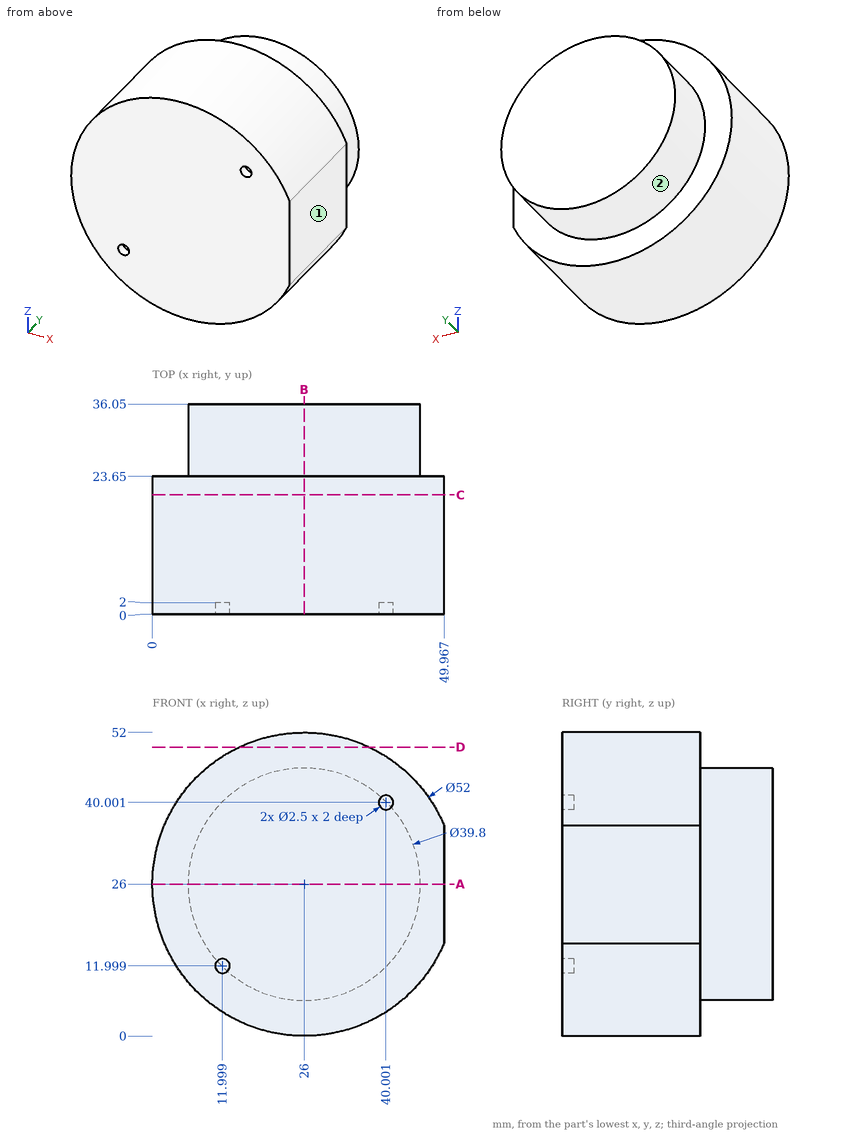
The drawing under review shows one solid part. Ordinate dimensions are in mm from its lowest x, y, z. A direction names the side the tool comes from. Coordinates: 2 decimals unless noted, no trailing zeros. Order: outer loops, then holes, each group sorted by start corner. A loop starts at its lowest first (then second) coordinate and runs counter-clockwise, first axis right, second up. Notation, with made-up numbers: (-34, -22.5) -> (-19, -22.5) arc R32 ccw to (-19, 16.5) -> close; hole circle Ø6 at (-3, 18.5). An arc over 180 degrees is marked (long way). Use CSV: the item, a comma, the result in double quotes. Start each with the question number.
Item 1: Insertion check: pin 1 (5 mm diameter, centred on x = 9.5, y = 19, fed in from +Z); pin 2 (10 mm diameter, centred on x = 40, y = 32.5, fed in from +Z); pin 3 (12 mm diameter, centred on y = 29, z = 45, fed in from -X). Each pin has a flat end and moves straight along its axis. Give the tip position at first contact, or say it passes through.
Item 2: We need section A-A, the plane z = 26. Give the boundary of the cut face in (x, y), then the cut area to 3 significant figures.
Item 3: Wall thickness on probe 1 along X at (y, z) = (17.5, 36); probe 2 along Y at (x, z) = (34, 6); probe 3 along X at (y, z) = (6, 26): over which ranges is each line inside the solid? List them lowest first.
Item 4: For the marked faces 1 and 2, list the 3-axis set-ups (+Z, -Z, +X, -X, +Y, -Y) from which the entire face can be reached by the end or side of a thin tool; tool diameter is ignored.
Item 5: We need section B-B, the plane x = 26. Give the boundary of the cut face in (y, z), then the cut area to 3 significant figures.
Item 6: We need section D-D, the plane z = 49.5. Give the boundary of the cut face in (x, y).
Item 7: We need section C-C, the plane y = 20.5. Give the boundary of the cut face in (x, z), then the cut area to 3 significant figures.
Derived:
1,pin 1,"stops at z = 47.91"
1,pin 2,"stops at z = 43.75"
1,pin 3,"stops at x = 5.73"
2,outline,"(0, 0) -> (49.97, 0) -> (49.97, 23.65) -> (45.9, 23.65) -> (45.9, 36.05) -> (6.1, 36.05) -> (6.1, 23.65) -> (0, 23.65) -> close"
2,area,"1,680 mm^2"
3,probe 1,"x = 2 to 49.97"
3,probe 2,"y = 0 to 23.65"
3,probe 3,"x = 0 to 49.97"
4,face 1,"+Z, -Z, +X, +Y, -Y"
4,face 2,"+Y"
5,outline,"(0, 0) -> (23.65, 0) -> (23.65, 6.1) -> (36.05, 6.1) -> (36.05, 45.9) -> (23.65, 45.9) -> (23.65, 52) -> (0, 52) -> close"
5,area,"1,720 mm^2"
6,outline,"(14.88, 0) -> (37.12, 0) -> (37.12, 23.65) -> (14.88, 23.65) -> close"
7,outline,"(49.97, 15.92) -> (49.97, 36.08) arc R26 ccw (long way) to start"
7,area,"2,100 mm^2"
